from build123d import *

# Parameters (mm, degrees)
SKETCH2_R           = 5
BOSS_EXTRUDE1_DEPTH = 10
SKETCH3_R           = 7.548336158
BOSS_EXTRUDE2_DEPTH = 5
BOSS_EXTRUDE3_START = 5
SKETCH4_R           = 7.548336158
BOSS_EXTRUDE3_DEPTH = 5


with BuildPart() as part:
    # Sketch2 → Boss-Extrude1 (new, symmetric)
    with BuildSketch(Plane.XY):
        Circle(SKETCH2_R)
    extrude(amount=BOSS_EXTRUDE1_DEPTH, both=True)

    # Sketch3 → Boss-Extrude2 (add)
    with BuildSketch(Plane.XY.offset(10)):
        Circle(SKETCH3_R)
    extrude(amount=BOSS_EXTRUDE2_DEPTH)

    # Sketch4 → Boss-Extrude3 (add)
    with BuildSketch(Plane(origin=(0, 0, -10), x_dir=(-1, 0, 0), z_dir=(0, 0, -1)).offset(BOSS_EXTRUDE3_START)):
        with Locations(Location((0, 0, 0), (0, 0, 180))):
            Circle(SKETCH4_R)
    extrude(amount=-BOSS_EXTRUDE3_DEPTH)


solid = part.part
For this review, take the finished solid that the model builds, in its own axes (mm). A direction names the side the tool comes from. Round coordinates to 2 decimals unless told otherwise and drop trailing zeros. Write each loop counter-clockwise with the first axis right and the second up, starting at its lowest first coordinate (ties: lowest second). Pieces come first, ordered by that corner, then holes. Notation, with made-up numbers: (49, 31) - (57, 31) arc R29 cw to (57, 53) - close; hole circle Ø7 at (-24, 32). An arc over 180 degrees is marked (long way). Use a Markdown table: item, result.
Q1. Machinability: for faces 1 (the flat face through (2, -5, 10)), 2 (the flat face through (0, 0, -15)), which of the approach directions +Z, -Z, +X, -X, +Y, -Y give a long, thin tool a straight path to every point of the face, cutting with its end or side? Answer none if there is none.
Derived:
| item | result |
|---|---|
| face 1 | none |
| face 2 | -Z, +X, -X, +Y, -Y |
Q2. We need section B-B (y = 6.75). Give the boundary of the cut face in (x, z), plus the area to 3 significant figures.
Derived:
| item | result |
|---|---|
| outline | (-3.38, -15) - (3.38, -15) - (3.38, -10) - (-3.38, -10) - close; (-3.38, 10) - (3.38, 10) - (3.38, 15) - (-3.38, 15) - close |
| area | 67.6 mm2 |
Q3. The part is to be moulded in two halves that separate along Z. For faces 3 (the cylindrical face through (-1.08, -4.88, 0.14)), 4 (the flat face through (0, 0, 15)), 5 (the cylindrical face through (-0.983, -7.484, -12.535)), say which applies: pulls with the +Z half, pulls with the -Z half, needs draft (parallel to the pull), parting line crosses it, or undercut.
Derived:
| item | result |
|---|---|
| face 3 | undercut |
| face 4 | pulls with the +Z half |
| face 5 | needs draft |
Q4. We need section D-D (z = 10.5). Give the boundary of the cut face in (x, y).
Derived:
| item | result |
|---|---|
| outline | circle Ø15.1 at (0, 0) |
Q5. Clearance check with flat-ended pins moving along their axes: pin 1 (6 mm diameter, centred on y = 4.5, z = -3, fed in from -X); pin 2 (6 mm diameter, centred on x = 1, z = 5.5, fed in from +Y); pin 3 (5 mm diameter, centred on x = -2, z = -2, fed in from -Y). State where each tip first meets the part, or that it passes through.
Derived:
| item | result |
|---|---|
| pin 1 | stops at x = -4.77 |
| pin 2 | stops at y = 5 |
| pin 3 | stops at y = -5 |
Q6. Wall thickness on line 1 along Z through (x, y) = (-6.5, 1); line 2 along X through (y, z) = (3, -11.75); line 3 along Y through (x, z) = (3.5, 6): over which ranges is each line inside the solid? List them lowest first.
Derived:
| item | result |
|---|---|
| line 1 | z = -15 to -10, 10 to 15 |
| line 2 | x = -6.93 to 6.93 |
| line 3 | y = -3.57 to 3.57 |
Q7. We need section A-A (y = 0). Give the boundary of the cut face in (x, z), plus the area to 3 significant figures.
Derived:
| item | result |
|---|---|
| outline | (-7.55, -15) - (7.55, -15) - (7.55, -10) - (5, -10) - (5, 10) - (7.55, 10) - (7.55, 15) - (-7.55, 15) - (-7.55, 10) - (-5, 10) - (-5, -10) - (-7.55, -10) - close |
| area | 351 mm2 |
